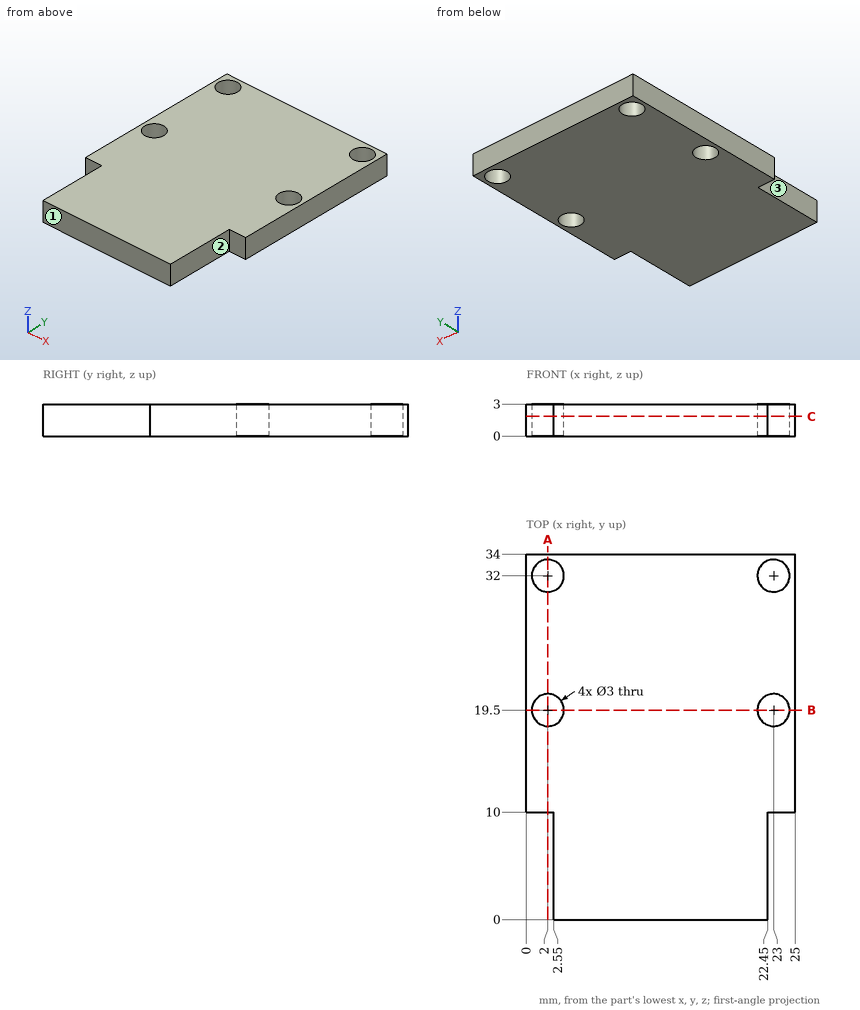
Design review of the part shown in the three views and the two pictorial views. Dimensions are in mm from the part's minimum x, y and z. A direction names the side the tool comes from. Round coordinates to 2 decimals unless told otherwise and drop trailing zeros. Order: outer loops, then holes, each group sorted by start corner. A loop starts at its lowest first (then second) coordinate and runs counter-clockwise, first axis right, second up. Notation, with made-up numbers: (53.5, 65) -> (72.5, 65) arc R23 cw to (72.5, 77) -> close; hole circle Ø4 at (-6.5, -33). An arc over 180 degrees is marked (long way). Write item = value, one per line. Start each with the question number.
1) Take a section at A-A on x = 2. State the section outline as (y, z) points.
2) To check wall thickness, follow line 1 (Y direction, x = 23, z = 0.7); line 2 (Y direction, x = 23.5, z = 0.55); line 3 (X direction, y = 4, z = 2.9). State the ranges of each line that lie inside material, in increasing order. Write a range as from..to.
3) Take a section at B-B on y = 19.5. State the section outline as (x, z) points, plus the area to 3 significant figures.
4) Take a section at C-C on z = 1.85. State the section outline as (x, y) points.
5) Insertion check: pin 1 (0.9 mm diameter, centred on y = 3, z = 1, fed in from -X); pin 2 (0.8 mm diameter, centred on x = 23, z = 1.5, fed in from -Y); pin 3 (2.5 mm diameter, centred on x = 23, y = 32, fed in from -Z); pin 4 (1.5 mm diameter, centred on y = 3.5, z = 2.5, fed in from +X). Each pin has a flat end and moves straight along its axis. Give the tip position at first contact, or say it passes through.
6) Tool access review of the marked faces 1, 2 and 3: name each direction out of +Z, -Z, +X, -X, +Y, -Y from which nothing blocks a thin tool from reaching the whole face with its end or side.
Verdict:
q1.outline = (10, 0) -> (18, 0) -> (18, 3) -> (10, 3) -> close; (21, 0) -> (30.5, 0) -> (30.5, 3) -> (21, 3) -> close; (33.5, 0) -> (34, 0) -> (34, 3) -> (33.5, 3) -> close
q2.line_1 = 10..18, 21..30.5, 33.5..34
q2.line_2 = 10..18.09, 20.91..30.59, 33.41..34
q2.line_3 = 2.55..22.45
q3.outline = (0, 0) -> (0.5, 0) -> (0.5, 3) -> (0, 3) -> close; (3.5, 0) -> (21.5, 0) -> (21.5, 3) -> (3.5, 3) -> close; (24.5, 0) -> (25, 0) -> (25, 3) -> (24.5, 3) -> close
q3.area = 57.0 mm2
q4.outline = (0, 10) -> (2.55, 10) -> (2.55, 0) -> (22.45, 0) -> (22.45, 10) -> (25, 10) -> (25, 34) -> (0, 34) -> close; hole circle Ø3 at (2, 19.5); hole circle Ø3 at (2, 32); hole circle Ø3 at (23, 19.5); hole circle Ø3 at (23, 32)
q5.pin_1 = 2.55
q5.pin_2 = 10
q5.pin_3 = through
q5.pin_4 = 22.45
q6.face_1 = +Z, -Z, +X, -X, -Y
q6.face_2 = +Z, -Z, +X, -Y
q6.face_3 = +Z, -Z, -X, -Y
